Work out the finished part from the listing and answer in its coordinate system (mm). A direction names the side the tool comes from. Coordinates: 2 decimals unless noted, no trailing zeros. Order: outer loops, then holes, each group sorted by start corner. A loop starts at its lowest first (then second) coordinate and runs counter-clockwise, first axis right, second up. Notation, with made-up numbers: (16.5, 86) - (74.5, 86) arc R25 cw to (74.5, 119) - close; hole circle Ø7 at (-9, 78.5). An arc over 180 degrees is marked (long way). Answer as a JSON object with one key per item and string values. Group by question number.
1) A tool of negligible diameter and unlimited length cuts with its end or side. For faces 1 (the face through (-13.096, 0.123, -6.746)), 2 (the face through (0, 12, 13)), from which of +Z, -Z, +X, -X, +Y, -Y can it reach the whole face along a straight path? Write none if from no direction.
2) Each of these flat-tipped pins is pushed along its axis until it touches: P1, Ø2, axis at y = 8.5, z = -2, coming from the -X side; P2, Ø12, axis at x = 0, z = 0, coming from the +Y side; P3, Ø5.5, axis at x = -20, y = -13.5, coming from the +Z side; P4, Ø6, axis at x = -2.5, z = -7.5, coming from the -Y side. Where does it stop, or does it pass through?
3) The mould has two halves that part along X. Classify faces 3 (the face through (6.29, 15.18, 8.47)), 4 (the face through (-13.933, 0.287, -8.353)), 5 (the face through (0, 0, -14)): released by +X, released by -X, zero draft, split by the parting line, or undercut.
4) Section C-C (y = 7) is taken. Give the vertices of the cut face in (x, z).
5) Section D-D (y = -6) is taken. Give the vertices of the cut face in (x, z).
6) Section B-B (z = 0) is taken. Give the vertices of the cut face in (x, y), plus the area to 3 significant figures.
7) Find the intervals of material crossed by line 1 along Y through (x, z) = (20, -12.85); line 2 along Y through (x, z) = (6.5, -10.25); line 3 along Y through (x, z) = (-3, 6.5), in increasing order.
8) Section A-A (x = -1) is taken. Give the vertices of the cut face in (y, z).
from build123d import *

# Parameters (mm, degrees)
SKETCH1_R            = 4.25
BOSS_EXTRUDE1_DEPTH  = 20.5
SKETCH2_W            = 14
SKETCH2_H            = 17.6
CUT_EXTRUDE1_DEPTH   = 29
SKETCH7_R            = 1
BOSS_EXTRUDE2_DEPTH  = 6
CUT_EXTRUDE6_DEPTH   = 3
SKETCH4_R            = 2
CUT_EXTRUDE2_DEPTH   = 7
SKETCH5_R            = 10
CUT_EXTRUDE3_DEPTH   = 8
SKETCH6_R            = 10
CUT_EXTRUDE4_DEPTH   = 8
FILLET1_R            = 1
CUT_EXTRUDE7_DEPTH   = 3
LPATTERN1_COUNT      = 2
LPATTERN1_PITCH      = 40
LPATTERN1_COUNT_DIR2 = 2
LPATTERN1_PITCH_DIR2 = 29


with BuildPart() as part:
    # Sketch1 → Boss-Extrude1 (new body, symmetric)
    with BuildSketch(Plane(origin=(0, 0, 0), x_dir=(1, 0, 0), z_dir=(0, 1, 0))):
        with BuildLine():
            Line((-12.931045729, -1.337182245), (-14, 9))
            Line((-14, 9), (-14, 15))
            Line((-14, 15), (14, 15))
            Line((14, 15), (14, 9))
            Line((14, 9), (12.931045729, -1.337182245))
            ThreePointArc((12.931045729, -1.337182245), (0, -13), (-12.931045729, -1.337182245))
        make_face()
        with Locations(Location((0, 0, 0), (0, 0, 270))):  # turned: the seam where the file's is
            Circle(SKETCH1_R, mode=Mode.SUBTRACT)
    extrude(amount=BOSS_EXTRUDE1_DEPTH, both=True)

    # Sketch2 → Cut-Revolve1 (revolve, cut)
    with BuildSketch(Plane(origin=(0, 0, 0), x_dir=(0, 0, -1), z_dir=(1, 0, 0))):
        with Locations((-7, 0)):
            Rectangle(SKETCH2_W, SKETCH2_H)
    revolve(axis=Axis((0, 0, 0), (0, 1, 0)), mode=Mode.SUBTRACT)

    # Sketch3 → Cut-Extrude1 (cut, through all)
    with BuildSketch(Plane(origin=(14, 0, 0), x_dir=(0, 0, -1), z_dir=(1, 0, 0))):
        Polygon((9, 20.5), (-13, 13.8), (-13, 20.5), align=None)
        Polygon((-13, -13.8), (9, -20.5), (-13, -20.5), align=None)
    extrude(amount=-CUT_EXTRUDE1_DEPTH, mode=Mode.SUBTRACT)

    # Sketch7 → Boss-Extrude2 (add)
    with BuildSketch(Plane(origin=(0, 0, -15), x_dir=(-1, 0, 0), z_dir=(0, 0, -1))):
        with BuildLine():
            Line((20, 20.5), (14, 20.5))
            Line((14, 20.5), (14, -20.5))
            Line((14, -20.5), (20, -20.5))
            ThreePointArc((20, -20.5), (25.516209879, -16.860387377), (24.340130723, -10.357142857))
            ThreePointArc((24.340130723, -10.357142857), (20.190457531, 0), (24.340130723, 10.357142857))
            ThreePointArc((24.340130723, 10.357142857), (25.516209879, 16.860387377), (20, 20.5))
        make_face()
        with Locations((20, -14.5)):
            Circle(SKETCH7_R, mode=Mode.SUBTRACT)
        with Locations((20, 14.5)):
            Circle(SKETCH7_R, mode=Mode.SUBTRACT)
        with BuildLine():
            Line((-20, -20.5), (-14, -20.5))
            Line((-14, -20.5), (-14, 20.5))
            Line((-14, 20.5), (-20, 20.5))
            ThreePointArc((-20, 20.5), (-25.516209879, 16.860387377), (-24.340130723, 10.357142857))
            ThreePointArc((-24.340130723, 10.357142857), (-20.190457531, 0), (-24.340130723, -10.357142857))
            ThreePointArc((-24.340130723, -10.357142857), (-25.516209879, -16.860387377), (-20, -20.5))
        make_face()
        with Locations((-20, 14.5)):
            Circle(SKETCH7_R, mode=Mode.SUBTRACT)
        with Locations((-20, -14.5)):
            Circle(SKETCH7_R, mode=Mode.SUBTRACT)
    extrude(amount=-BOSS_EXTRUDE2_DEPTH)

    # Sketch8 → Cut-Extrude6 (cut)
    with BuildSketch(Plane.XY.offset(-9)):
        Polygon((-17.15, 12.854551733), (-17.15, 16.145448267), (-20, 17.790896534), (-22.85, 16.145448267), (-22.85, 12.854551733), (-20, 11.209103466), align=None)
        Polygon((-17.15, -12.854551733), (-20, -11.209103466), (-22.85, -12.854551733), (-22.85, -16.145448267), (-20, -17.790896534), (-17.15, -16.145448267), align=None)
        Polygon((22.85, -12.854551733), (20, -11.209103466), (17.15, -12.854551733), (17.15, -16.145448267), (20, -17.790896534), (22.85, -16.145448267), align=None)
        Polygon((22.85, 12.854551733), (22.85, 16.145448267), (20, 17.790896534), (17.15, 16.145448267), (17.15, 12.854551733), (20, 11.209103466), align=None)
    extrude(amount=-CUT_EXTRUDE6_DEPTH, mode=Mode.SUBTRACT)

    # Sketch4 → Cut-Extrude2 (cut)
    with BuildSketch(Plane(origin=(0, 0, -15), x_dir=(-1, 0, 0), z_dir=(0, 0, -1))):
        with Locations((-20, 14.5)):
            Circle(SKETCH4_R)
        with Locations((20, 14.5)):
            Circle(SKETCH4_R)
        with Locations((-20, -14.5)):
            Circle(SKETCH4_R)
        with Locations((20, -14.5)):
            Circle(SKETCH4_R)
    extrude(amount=-CUT_EXTRUDE2_DEPTH, mode=Mode.SUBTRACT)

    # Sketch5 → Cut-Extrude3 (cut)
    with BuildSketch(Plane(origin=(0, 20.5, 0), x_dir=(1, 0, 0), z_dir=(0, 1, 0))):
        with Locations(Location((0, 0, 0), (0, 0, 270))):  # turned: the seam where the file's is
            Circle(SKETCH5_R)
    extrude(amount=-CUT_EXTRUDE3_DEPTH, mode=Mode.SUBTRACT)

    # Sketch6 → Cut-Extrude4 (cut)
    with BuildSketch(Plane.XZ.offset(20.5)):
        with Locations(Location((0, 0, 0), (0, 0, 90))):  # turned: the seam where the file's is
            Circle(SKETCH6_R)
    extrude(amount=-CUT_EXTRUDE4_DEPTH, mode=Mode.SUBTRACT)

    # Fillet1
    fillet1_edges = [part.edges().sort_by_distance(p)[0] for p in [
        (13.465522864, 0, -3.831408877),
        (-13.465522864, 0, -3.831408877),
    ]]
    fillet(fillet1_edges, radius=FILLET1_R)

    # Sketch9 → Cut-Extrude7 (cut)
    with BuildSketch(Plane.XY.offset(-9)):
        with BuildLine():
            ThreePointArc((-23.35, 16.434123402), (-22.85, 14.5), (-23.35, 12.565876598))
            ThreePointArc((-23.35, 12.565876598), (-21.425, 12.031827599), (-20, 10.631753196))
            ThreePointArc((-20, 10.631753196), (-18.575, 12.031827599), (-16.65, 12.565876598))
            ThreePointArc((-16.65, 12.565876598), (-17.15, 14.5), (-16.65, 16.434123402))
            ThreePointArc((-16.65, 16.434123402), (-18.575, 16.968172401), (-20, 18.368246804))
            ThreePointArc((-20, 18.368246804), (-21.425, 16.968172401), (-23.35, 16.434123402))
        make_face()
    cut_extrude7 = extrude(amount=-CUT_EXTRUDE7_DEPTH, mode=Mode.SUBTRACT)

    # LPattern1: Cut-Extrude7 2 × 2
    with Locations(*[(i * LPATTERN1_PITCH, -j * LPATTERN1_PITCH_DIR2, 0) for i in range(LPATTERN1_COUNT) for j in range(LPATTERN1_COUNT_DIR2) if (i, j) != (0, 0)]):
        add(cut_extrude7, mode=Mode.SUBTRACT)


solid = part.part
Report:
{
 "1": {"face 1": "+Z", "face 2": "+Z, +Y, -Y"},
 "2": {"P1": "stops at x = -13.37", "P2": "stops at y = 12.5", "P3": "stops at z = -9", "P4": "stops at y = -20.5"},
 "3": {"face 3": "zero draft", "face 4": "released by -X", "face 5": "undercut"},
 "4": {"outline": "(-21.92, -15) - (21.92, -15) - (21.92, -9) - (14, -9) - (13.86, -7.62) arc R1 ccw to (12, -7.2) arc R14 cw to (-12, -7.2) arc R1 ccw to (-13.86, -7.62) - (-14, -9) - (-21.92, -9) - close"},
 "5": {"outline": "(-21.44, -15) - (21.44, -15) - (21.44, -9) - (14, -9) - (13.86, -7.62) arc R1 ccw to (12, -7.2) arc R14 cw to (-12, -7.2) arc R1 ccw to (-13.86, -7.62) - (-14, -9) - (-21.44, -9) - close"},
 "6": {"outline": "(-13.07, -17.76) - (-10, -17.76) - (-10, -12.5) - (-4.25, -12.5) - (-4.25, -8.8) - (-13.07, -8.8) - close; (-13.07, 8.8) - (-4.25, 8.8) - (-4.25, 12.5) - (-10, 12.5) - (-10, 17.76) - (-13.07, 17.76) - close; (4.25, -12.5) - (10, -12.5) - (10, -17.76) - (13.07, -17.76) - (13.07, -8.8) - (4.25, -8.8) - close; (4.25, 8.8) - (13.07, 8.8) - (13.07, 17.76) - (10, 17.76) - (10, 12.5) - (4.25, 12.5) - close", "area": "195 mm²"},
 "7": {"line 1": "y = -20.5 to -16.5, -12.5 to 12.5, 16.5 to 20.5", "line 2": "y = -20.5 to -8.8, 8.8 to 20.5", "line 3": "y = -12.5 to -8.8, 8.8 to 12.5"},
 "8": {"outline": "(-20.5, -15) - (20.5, -15) - (20.5, -9.95) - (12.5, -9.95) - (12.5, -4.13) - (8.8, -4.13) - (8.8, -13.96) - (-8.8, -13.96) - (-8.8, -4.13) - (-12.5, -4.13) - (-12.5, -9.95) - (-20.5, -9.95) - close; (-14.73, 9.95) - (-12.5, 9.95) - (-12.5, 4.13) - (-8.8, 4.13) - (-8.8, 12.96) - (-13.81, 12.96) - close; (8.8, 4.13) - (12.5, 4.13) - (12.5, 9.95) - (14.73, 9.95) - (13.81, 12.96) - (8.8, 12.96) - close"}
}
